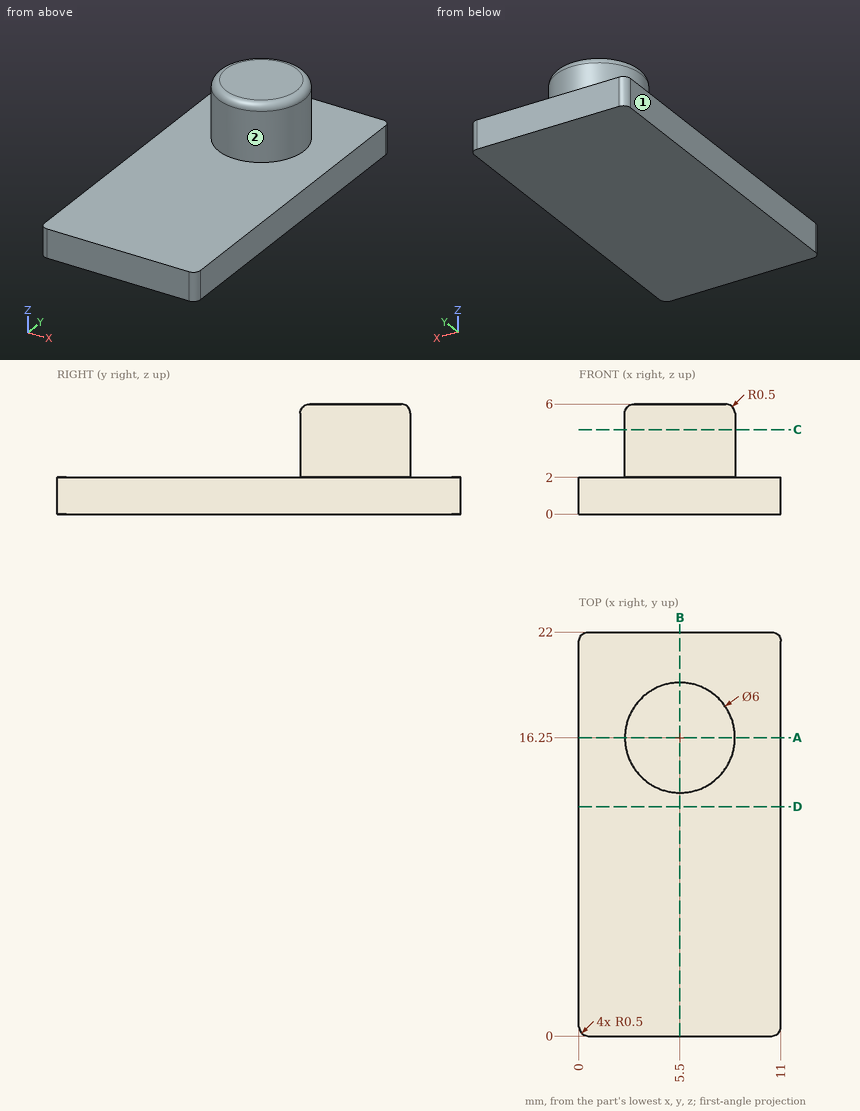
For this review, use the dimensioned drawing (mm, ordinates from the lowest corner) and the shaded views. A direction names the side the tool comes from. Give positions to 0.01 mm unless a question says otherwise; leave off trailing zeros. Loops run counter-clockwise (first coordinate to the right, second up) from the corner with the lowest first, then second, coordinate; pieces in that order, holes last.
Item 1: Insertion check: pin 1 (2 mm diameter, centred on y = 15, z = 4.5, fed in from -X). The pin has a flat end and moves straight along its axis. Give the tip position at first contact, or say it passes through.
Item 2: Tool access review of the marked faces 1 and 2: name each direction out of +Z, -Z, +X, -X, +Y, -Y from which nothing blocks a thin tool from reaching the whole face with its end or side.
Item 3: For line 1 along Z through (x, y) = (4.25, 1.75); line 2 along Y through (x, z) = (5.5, 3.1); line 3 along X through (y, z) = (18, 2.55), list the stretches that pass through material, from the lowest coordinate up.
Item 4: Take a section at A-A, the plane y = 16.25. State the section outline as (x, z) points.
Item 5: Take a section at C-C, the plane z = 4.6. State the section outline as (x, y) points.
Item 6: Take a section at D-D, the plane y = 12.5. State the section outline as (x, z) points, and give its area (3 significant figures).
Item 7: Take a section at B-B, the plane x = 5.5. State the section outline as (y, z) points.
Calculated:
1. pin 1: stops at x = 2.51
2. face 1: +Z, -Z, -X, +Y, -Y
2. face 2: +Z
3. line 1: z = 0 to 2
3. line 2: y = 13.25 to 19.25
3. line 3: x = 3.06 to 7.94
4. outline: (0, 0) - (11, 0) - (11, 2) - (8.5, 2) - (8.5, 5.5) arc R0.5 ccw to (8, 6) - (3, 6) arc R0.5 ccw to (2.5, 5.5) - (2.5, 2) - (0, 2) - close
5. outline: circle Ø6 at (5.5, 16.25)
6. outline: (0, 0) - (11, 0) - (11, 2) - (0, 2) - close
6. area: 22.0 mm2
7. outline: (0, 0) - (22, 0) - (22, 2) - (19.25, 2) - (19.25, 5.5) arc R0.5 ccw to (18.75, 6) - (13.75, 6) arc R0.5 ccw to (13.25, 5.5) - (13.25, 2) - (0, 2) - close
